```python
from build123d import *

# Parameters (mm, degrees)
SKETCH1_W           = 1000
SKETCH1_H           = 1200
BOSS_EXTRUDE1_DEPTH = 20
SKETCH2_W           = 1000
SKETCH2_H           = 1200
SKETCH2_W_2         = 983.333333334
SKETCH2_H_2         = 1180
BOSS_EXTRUDE2_DEPTH = 600
SKETCH3_W           = 227.751399754
SKETCH3_H           = 224.45065483
SKETCH3_H_2         = 247.555869298
SKETCH3_H_3         = 212.898047596
SKETCH3_W_2         = 244.255124374
SKETCH3_H_4         = 242.604751912
SKETCH3_H_5         = 207.946930211
SKETCH3_W_3         = 488.510248749
SKETCH3_H_6         = 320.94890349
BOSS_EXTRUDE3_DEPTH = 400
SKETCH13_R          = 50
CUT_EXTRUDE1_DEPTH  = 1441.277750991


with BuildPart() as part:
    # Sketch1 → Boss-Extrude1 (new body)
    with BuildSketch(Plane(origin=(0, 0, 0), x_dir=(1, 0, 0), z_dir=(0, 1, 0))):
        Rectangle(SKETCH1_W, SKETCH1_H)
    extrude(amount=BOSS_EXTRUDE1_DEPTH)

    # Sketch2 → Boss-Extrude2 (add)
    with BuildSketch(Plane(origin=(0, 20, 0), x_dir=(1, 0, 0), z_dir=(0, 1, 0))):
        Rectangle(SKETCH2_W, SKETCH2_H)
        Rectangle(SKETCH2_W_2, SKETCH2_H_2, mode=Mode.SUBTRACT)
    extrude(amount=BOSS_EXTRUDE2_DEPTH)

    # Sketch3 → Boss-Extrude3 (add)
    with BuildSketch(Plane(origin=(0, 20, 0), x_dir=(1, 0, 0), z_dir=(0, 1, 0))):
        with Locations((-267.360338842, 405.166439418)):
            Rectangle(SKETCH3_W, SKETCH3_H)
        with Locations((310.270022854, 405.166439418)):
            Rectangle(SKETCH3_W, SKETCH3_H_2)
        with Locations((-267.360338842, 0)):
            Rectangle(SKETCH3_W, SKETCH3_H_3)
        with Locations((310.270022854, 0)):
            Rectangle(SKETCH3_W_2, SKETCH3_H_4)
        with Locations((-267.360338842, -357.305638021)):
            Rectangle(SKETCH3_W, SKETCH3_H_5)
        with Locations((209.597302673, -395.264204646)):
            Rectangle(SKETCH3_W_3, SKETCH3_H_6)
    extrude(amount=BOSS_EXTRUDE3_DEPTH)

    # Sketch13 → Cut-Extrude1 (cut, through all)
    with BuildSketch(Plane.XY.offset(600)):
        with Locations((-359.206066916, 536.564881977)):
            Circle(SKETCH13_R)
        with Locations((-102.023024923, 530.188442919)):
            Circle(SKETCH13_R)
        with Locations((170.038374872, 530.188442919)):
            Circle(SKETCH13_R)
        with Locations((397.464701262, 536.564881977)):
            Circle(SKETCH13_R)
    extrude(amount=-CUT_EXTRUDE1_DEPTH, mode=Mode.SUBTRACT)


solid = part.part
```
Geometry: final body of the model. Coordinates: model frame, mm. A direction names the side the tool comes from. Coordinates: 2 decimals unless noted, no trailing zeros. Loops run counter-clockwise (first coordinate to the right, second up) from the corner with the lowest first, then second, coordinate; pieces in that order, holes last. Notation, with made-up numbers: (9.5, 82.5) -> (40.5, 82.5) arc R34 cw to (40.5, 117.5) -> close; hole circle Ø2 at (7.25, 32.5). An arc over 180 degrees is marked (long way). Use a Markdown table: item, result. Add a question column.
(1) Mould query, pull axis Z, two halves, no side actions, for faces 1 (the flat face through (309, 217, 121.302)), 2 (the cylindrical face through (159.199, 481.377, 595.07)). Classes: pulls with the +Z half, pulls with the -Z half, needs draft (parallel to the pull), parting line crosses it, or undercut.
(2) Section query B-B, the plane z = -71. Return loops of the section in (x, y).
(3) Access query for faces 3 (the flat face through (-500, 306, 8)), 4 (the flat face through (309, 217, -281.389)). Directions: +Z, -Z, +X, -X, +Y, -Y. A direction counts if a zero-diameter tool reaches every point of the face in a straight line with its end or side. Return the directions, or none.
(4) Section query C-C, the plane x = -432.5. Return loops of the section in (y, z).
(5) Section query A-A, the plane y = 320. State how many separate pieces and enclosed holes the cut face has, plus the area to 3 significant figures.
(6) Section query D-D, the plane x = -241. Return loops of the section in (y, z), plus the area to 3 significant figures.
(7) Pin query (flat end, axial travel): pin 1 Ø1.5 at (x, z) = (351, -412) entering from +Y. Return the tip coordinate at first contact, or that it passes through.
(8) Line query: line 1 along X through (y, z) = (269.5, 404); line 2 along X through (y, z) = (87.5, -455); line 3 along Z through (x, y) = (243, 381.5). Output: solid intervals per line, ascending.
Answer:
| question | item | result |
|---|---|---|
| 1 | face 1 | undercut |
| 1 | face 2 | needs draft |
| 2 | outline | (-500, 0) -> (500, 0) -> (500, 620) -> (491.67, 620) -> (491.67, 20) -> (432.4, 20) -> (432.4, 420) -> (188.14, 420) -> (188.14, 20) -> (-153.48, 20) -> (-153.48, 420) -> (-381.24, 420) -> (-381.24, 20) -> (-491.67, 20) -> (-491.67, 620) -> (-500, 620) -> close |
| 3 | face 3 | +Z, -Z, -X, +Y, -Y |
| 3 | face 4 | +Y |
| 4 | outline | (0, -600) -> (620, -600) -> (620, -590) -> (20, -590) -> (20, 590) -> (620, 590) -> (620, 600) -> (0, 600) -> close |
| 5 | separate pieces | 7 |
| 5 | enclosed holes | 1 |
| 5 | area | 459,000 mm^2 |
| 6 | outline | (0, -600) -> (620, -600) -> (620, -590) -> (20, -590) -> (20, -517.39) -> (420, -517.39) -> (420, -292.94) -> (20, -292.94) -> (20, -106.45) -> (420, -106.45) -> (420, 106.45) -> (20, 106.45) -> (20, 253.33) -> (420, 253.33) -> (420, 461.28) -> (20, 461.28) -> (20, 590) -> (620, 590) -> (620, 600) -> (0, 600) -> close |
| 6 | area | 294,000 mm^2 |
| 7 | pin 1 | stops at y = 420 |
| 8 | line 1 | x = -500 to -491.67, -381.24 to -153.48, -34.66 to 453.85, 491.67 to 500 |
| 8 | line 2 | x = -500 to -491.67, -381.24 to -153.48, 196.39 to 424.15, 491.67 to 500 |
| 8 | line 3 | z = -600 to -590, -528.94 to -281.39, -121.3 to 121.3, 234.79 to 555.74, 590 to 600 |
